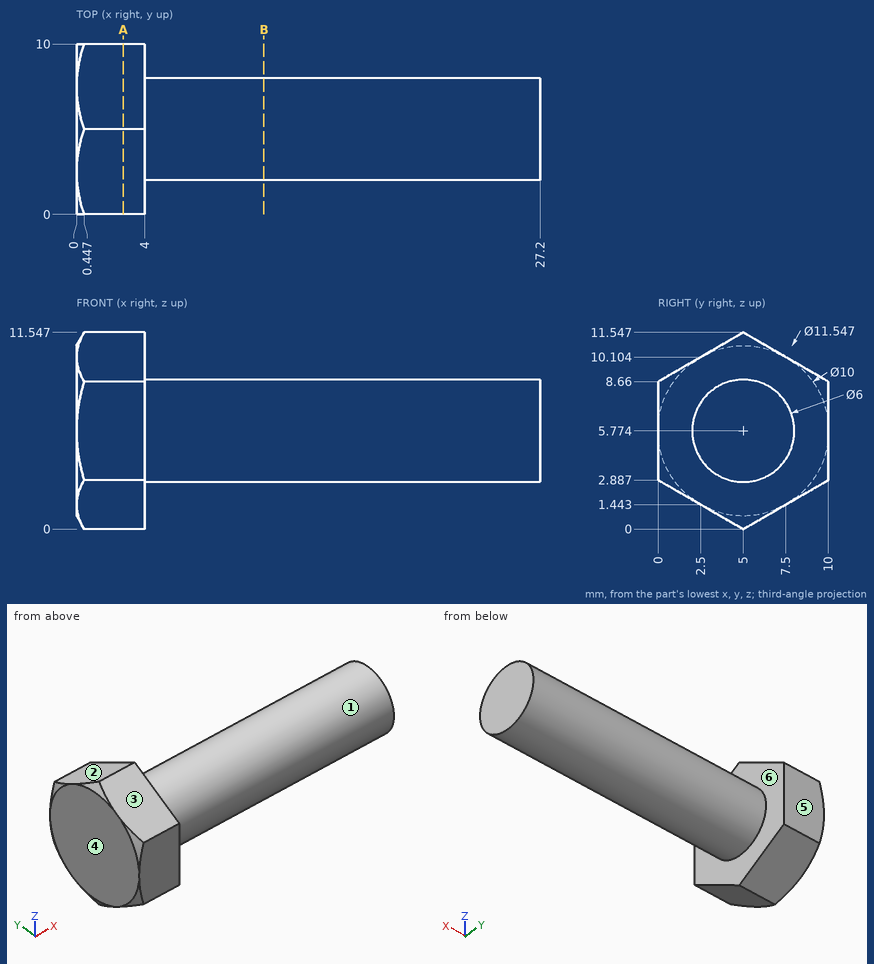
Geometry check sheet. Reference: drawing and pictorial views, mm from the part's lowest x, y, z. A direction names the side the tool comes from. Give positions to 0.01 mm unless a question says otherwise; leave off trailing zeros. Order: outer loops, then holes, each group sorted by start corner. A loop starts at its lowest first (then second) coordinate and runs counter-clockwise, first axis right, second up. Notation, with made-up numbers: (-39, 31) -> (2, 31) arc R24 ccw to (2, 47) -> close; hole circle Ø7 at (54.25, 45.5). An arc over 180 degrees is marked (long way). Use CSV: the item, a comma, the result in double quotes. Start each with the question number.
1) Material ranges on line 1 (X direction, y = 2.75, z = 1.75); line 2 (Y direction, x = 6.5, z = 3.5) (1 decimal); line 3 (X direction, y = 9.75, z = 8.5) (1 decimal), recorded low to high. Write a range as from..to.
2) Go/stop test with flat-tipped pins: P1, Ø5, axis at x = 11, y = 2.5, coming from the +Z side; P2, Ø3, axis at x = 22, y = 6.5, coming from the -Z side; P3, Ø6, axis at x = 10.5, z = 1.5, coming from the -Y side. Record where each tip stops, or that it passes through.
3) Sectioned sample at A-A, the plane x = 2.75. Record the boundary of the cut face in (y, z), plus the area to 3 significant figures.
4) Mould release check, pull along Y, two halves, no side actions. Record for the marked faces 1, 2, 3 and 4: released by +Y, released by -Y, zero draft, split by the parting line, or undercut.
5) Sectioned sample at B-B, the plane x = 11. Record the boundary of the cut face in (y, z), plus the area to 3 significant figures.
6) Set-up check for the marked faces 5 and 6: record each of +Z, -Z, +X, -X, +Y, -Y from which the full face is reachable in a straight line by a thin tool's end or side.
Recorded:
1,line 1,"0..4"
1,line 2,"3..7"
1,line 3,"0.3..4"
2,P1,"z = 8.77"
2,P2,"z = 2.77"
2,P3,"y = 2.28"
3,outline,"(0, 2.89) -> (5, 0) -> (10, 2.89) -> (10, 8.66) -> (5, 11.55) -> (0, 8.66) -> close"
3,area,"86.6 mm2"
4,face 1,"split by the parting line"
4,face 2,"released by +Y"
4,face 3,"released by -Y"
4,face 4,"zero draft"
5,outline,"circle Ø6 at (5, 5.77)"
5,area,"28.3 mm2"
6,face 5,"+Z, -Z, +X, -X, +Y"
6,face 6,"+X"
